Here's how the part is built. I have some questions about the finished solid (model axes, mm). A direction names the side the tool comes from. Coordinates: 2 decimals unless noted, no trailing zeros.
Item 1: I'm going to push flat-ended pins straight in: P1, Ø12, axis at y = 8.5, z = -104, coming from the -X side; P2, Ø1, axis at x = 97.5, y = 4.5, coming from the -Z side; P3, Ø6.5, axis at x = 75.8, z = -68.25, coming from the +Y side; P4, Ø4, axis at y = 14.5, z = -28.5, coming from the +X side. Where does each tip first touch, or does it pass through?
Item 2: I want a section at A-A (y = 4). Count the separate pieces of the cut face and the enclosed holes in it, and give its area (3 significant figures).
Item 3: For faces 1 (the face through (92.795, 11.661, -53.794)), 2 (the face through (66, 20.4, -89)), 3 (the face through (95.69, 9.86, -54.78)), 4 (the face through (99.09, 20.03, -31.79)), which set-ups out of +Z, -Z, +X, -X, +Y, -Y let a thin tool reach every point of the face, with its end or its side?
Item 4: Please list where these lines run through material, in increasing order: line 1 (Y direction, x = 95, z = -2); line 2 (Z direction, x = 76, y = 18.5); line 3 (Z direction, x = 90, y = 16.5).
from build123d import *

# Parameters (mm, degrees)
BOSS_EXTRUDE1_DEPTH      = 23
SKETCH2_W                = 100.4
SKETCH2_H                = 20.4
CUT_EXTRUDE2_DEPTH       = 20.4
CUT_EXTRUDE3_DEPTH       = 20
SKETCH7_R                = 2.3
CUT_EXTRUDE6_DEPTH       = 10
SKETCH8_R                = 2.3
CUT_EXTRUDE7_DEPTH       = 10
FILLET3_R                = 35
CUT_EXTRUDE11_DEPTH      = 200.759855827
CUT_EXTRUDE11_DEPTH_BACK = 200.759855827
CUT_EXTRUDE10_DEPTH      = 20
BOSS_EXTRUDE3_DEPTH      = 6
BOSS_EXTRUDE4_DEPTH      = 17
CUT_EXTRUDE14_DEPTH      = 17
SKETCH30_R               = 1.5
CUT_EXTRUDE15_DEPTH      = 200.158228552
SKETCH31_R               = 2.9
CUT_EXTRUDE17_DEPTH      = 3
SKETCH32_R               = 2.3
CUT_EXTRUDE18_DEPTH      = 10
SKETCH33_R               = 2.3
CUT_EXTRUDE19_DEPTH      = 10
SKETCH34_R               = 2.3
CUT_EXTRUDE20_DEPTH      = 149.465956609
SKETCH35_R               = 4
CUT_EXTRUDE21_DEPTH      = 154.248582194
SKETCH36_R               = 2.1
CUT_EXTRUDE22_DEPTH      = 5
SKETCH37_R               = 2.1
CUT_EXTRUDE23_DEPTH      = 5
SKETCH38_R               = 2.3
CUT_EXTRUDE24_DEPTH      = 10
CHAMFER1_SIZE            = 1


with BuildPart() as part:
    # Sketch1 → Boss-Extrude1 (new body)
    with BuildSketch(Plane(origin=(0, 0, 0), x_dir=(1, 0, 0), z_dir=(0, 1, 0))):
        Polygon((0, 0), (150, 0), (75, 129.903810568), align=None)
    extrude(amount=BOSS_EXTRUDE1_DEPTH)

    # Sketch2 → Cut-Extrude2 (cut)
    with BuildSketch(Plane(origin=(0, 0, 0), x_dir=(1, 0, 0), z_dir=(0, 1, 0))):
        Polygon((108.923840175, 138.261625339), (58.723840175, 51.312674799), (41.056921938, 61.512674799), (91.256921938, 148.461625339), align=None)
        with Locations((124, 15)):
            Rectangle(SKETCH2_W, SKETCH2_H)
    extrude(amount=CUT_EXTRUDE2_DEPTH, mode=Mode.SUBTRACT)

    # Sketch4 → Cut-Extrude3 (cut)
    with BuildSketch(Plane(origin=(0, 0, 0), x_dir=(1, 0, 0), z_dir=(0, 1, 0))):
        Polygon((58.515583945, 45.561933634), (40.848665708, 35.361933634), (51.048665708, 17.695015397), (68.715583945, 27.895015397), align=None)
    extrude(amount=CUT_EXTRUDE3_DEPTH, mode=Mode.SUBTRACT)

    # Sketch7 → Cut-Extrude6 (cut)
    with BuildSketch(Plane(origin=(0, 0, 0), x_dir=(-0.4999999999999978, 0, 0.86602540378444), z_dir=(-0.86602540378444, 0, -0.4999999999999978))):
        with Locations((-130, 10)):
            Circle(SKETCH7_R)
        with Locations((-95, 10)):
            Circle(SKETCH7_R)
    extrude(amount=-CUT_EXTRUDE6_DEPTH, mode=Mode.SUBTRACT)

    # Sketch8 → Cut-Extrude7 (cut)
    with BuildSketch(Plane.XY):
        with Locations((130, 10)):
            Circle(SKETCH8_R)
        with Locations((95, 10)):
            Circle(SKETCH8_R)
    extrude(amount=-CUT_EXTRUDE7_DEPTH, mode=Mode.SUBTRACT)

    # Fillet3
    fillet3_edges = [part.edges().sort_by_distance(p)[0] for p in [
        (0, 11.5, 0),
    ]]
    fillet(fillet3_edges, radius=FILLET3_R)

    # Sketch22 → Cut-Extrude11 (cut, two sides: drawn at the far end of the back side and taken through both)
    with BuildSketch(Plane.XZ.offset(-CUT_EXTRUDE11_DEPTH_BACK)):
        Polygon((76.257198908, -28.438657049), (62.757198908, -51.821342951), (86.13988481, -65.321342951), (99.63988481, -41.938657049), align=None)
    extrude(amount=CUT_EXTRUDE11_DEPTH + CUT_EXTRUDE11_DEPTH_BACK, mode=Mode.SUBTRACT)

    # Sketch21 → Cut-Extrude10 (cut)
    with BuildSketch(Plane.XZ):
        Polygon((132.679491924, -30), (109.996773286, -30), (80.979148757, -80.26), (92.320508076, -99.903810568), align=None)
    extrude(amount=-CUT_EXTRUDE10_DEPTH, mode=Mode.SUBTRACT)

    # Sketch27 → Boss-Extrude3 (add)
    with BuildSketch(Plane(origin=(0, 23, 0), x_dir=(1, 0, 0), z_dir=(0, 1, 0))):
        Polygon((76.257198908, 28.438657049), (62.757198908, 51.821342951), (68.819376734, 55.321342951), (82.319376734, 31.938657049), align=None)
    extrude(amount=-BOSS_EXTRUDE3_DEPTH)

    # Sketch28 → Boss-Extrude4 (add)
    with BuildSketch(Plane.XZ.offset(-17)):
        Polygon((74.257198908, -31.902758664), (64.757198908, -48.357241336), (70.819376734, -51.857241336), (80.319376734, -35.402758664), align=None)
    extrude(amount=BOSS_EXTRUDE4_DEPTH)

    # Sketch29 → Cut-Extrude14 (cut)
    with BuildSketch(Plane.XZ):
        Polygon((77.819376734, -39.732885683), (71.757198908, -36.232885683), (67.257198908, -44.027114317), (73.319376734, -47.527114317), align=None)
    extrude(amount=-CUT_EXTRUDE14_DEPTH, mode=Mode.SUBTRACT)

    # Sketch30 → Cut-Extrude15 (cut, through all)
    with BuildSketch(Plane.XZ.offset(-17)):
        with Locations(Location((72.971300523, -42.13, 0), (0, 0, 270))):
            Circle(SKETCH30_R)
    extrude(amount=-CUT_EXTRUDE15_DEPTH, mode=Mode.SUBTRACT)

    # Sketch31 → Cut-Extrude17 (cut)
    with BuildSketch(Plane(origin=(0, 23, 0), x_dir=(1, 0, 0), z_dir=(0, 1, 0))):
        with Locations(Location((72.971300523, 42.13, 0), (0, 0, 270))):
            Circle(SKETCH31_R)
    extrude(amount=-CUT_EXTRUDE17_DEPTH, mode=Mode.SUBTRACT)

    # Sketch32 → Cut-Extrude18 (cut)
    with BuildSketch(Plane(origin=(0, 0, -30), x_dir=(-1, 0, 0), z_dir=(0, 0, -1))):
        with Locations((-121.338132605, 10)):
            Circle(SKETCH32_R)
    extrude(amount=-CUT_EXTRUDE18_DEPTH, mode=Mode.SUBTRACT)

    # Sketch33 → Cut-Extrude19 (cut)
    with BuildSketch(Plane(origin=(25.980762114, 0, 15), x_dir=(0.4999999999999997, 0, -0.8660254037844388), z_dir=(0.8660254037844389, 0, 0.49999999999999983))):
        with Locations((121.338132605, 10)):
            Circle(SKETCH33_R)
    extrude(amount=-CUT_EXTRUDE19_DEPTH, mode=Mode.SUBTRACT)

    # Sketch34 → Cut-Extrude20 (cut, through all)
    with BuildSketch(Plane(origin=(45.948665708, 0, -26.528474516), x_dir=(-0.5000000000000001, 0, -0.8660254037844386), z_dir=(0.8660254037844386, 0, -0.5000000000000001))):
        with Locations((0, 10)):
            Circle(SKETCH34_R)
    extrude(amount=-CUT_EXTRUDE20_DEPTH, mode=Mode.SUBTRACT)

    # Sketch35 → Cut-Extrude21 (cut, through all)
    with BuildSketch(Plane(origin=(41.618538689, 0, -24.028474516), x_dir=(-0.5000000000000001, 0, -0.8660254037844386), z_dir=(0.8660254037844386, 0, -0.5000000000000001))):
        with Locations((0, 10)):
            Circle(SKETCH35_R)
    extrude(amount=-CUT_EXTRUDE21_DEPTH, mode=Mode.SUBTRACT)

    # Sketch36 → Cut-Extrude22 (cut)
    with BuildSketch(Plane(origin=(0, 23, 0), x_dir=(1, 0, 0), z_dir=(0, 1, 0))):
        with Locations(Location((38.97114317, 22.5, 0), (0, 0, 270))):
            Circle(SKETCH36_R)
    extrude(amount=-CUT_EXTRUDE22_DEPTH, mode=Mode.SUBTRACT)

    # Sketch37 → Cut-Extrude23 (cut)
    with BuildSketch(Plane(origin=(0, 23, 0), x_dir=(1, 0, 0), z_dir=(0, 1, 0))):
        with Locations(Location((97.007764662, 31.519733426, 0), (0, 0, 270))):
            Circle(SKETCH37_R)
        with Locations(Location((75.800772199, 68.251321849, 0), (0, 0, 270))):
            Circle(SKETCH37_R)
    extrude(amount=-CUT_EXTRUDE23_DEPTH, mode=Mode.SUBTRACT)

    # Sketch38 → Cut-Extrude24 (cut)
    with BuildSketch(Plane.XZ.offset(-20.4)):
        with Locations(Location((88.8, -15, 0), (0, 0, 270))):
            Circle(SKETCH38_R)
        with Locations(Location((123.8, -15, 0), (0, 0, 270))):
            Circle(SKETCH38_R)
        with Locations(Location((57.390381057, -69.403055856, 0), (0, 0, 270))):
            Circle(SKETCH38_R)
        with Locations(Location((74.890381057, -99.713944989, 0), (0, 0, 270))):
            Circle(SKETCH38_R)
    extrude(amount=-CUT_EXTRUDE24_DEPTH, mode=Mode.SUBTRACT)

    # Chamfer1
    chamfer1_edges = [part.edges().sort_by_distance(p)[0] for p in [
        (38.97114317, 23, -24.6),
        (97.007764662, 23, -33.619733426),
        (75.800772199, 23, -70.351321849),
    ]]
    chamfer(chamfer1_edges, length=CHAMFER1_SIZE)


solid = part.part
Answer:
1. P1: stops at x = 56.58
1. P2: stops at z = -52.51
1. P3: stops at y = 23
1. P4: stops at x = 134.7
2. separate pieces: 1
2. enclosed holes: 2
2. area: 3,710 mm2
3. face 1: +Y, -Y
3. face 2: -Y
3. face 3: +X, -Y
3. face 4: +Y
4. line 1: y = 0 to 7.7, 12.3 to 23
4. line 2: z = -128.17 to -122.04, -81.24 to -70.34, -66.16 to -59.47, -42.88 to -25.2, -4.8 to 0
4. line 3: z = -103.92 to -95.88, -64.64 to -58.64, -36.37 to -25.2, -4.8 to 0
